Check sheet for the drawn part. Datum: minimum x, y, z corner. Units: mm. Give positions to 0.01 mm unless a question says otherwise; leave off trailing zeros. Loops run counter-clockwise (first coordinate to the right, second up) from the corner with the lowest first, then second, coordinate; pieces in that order, holes last.
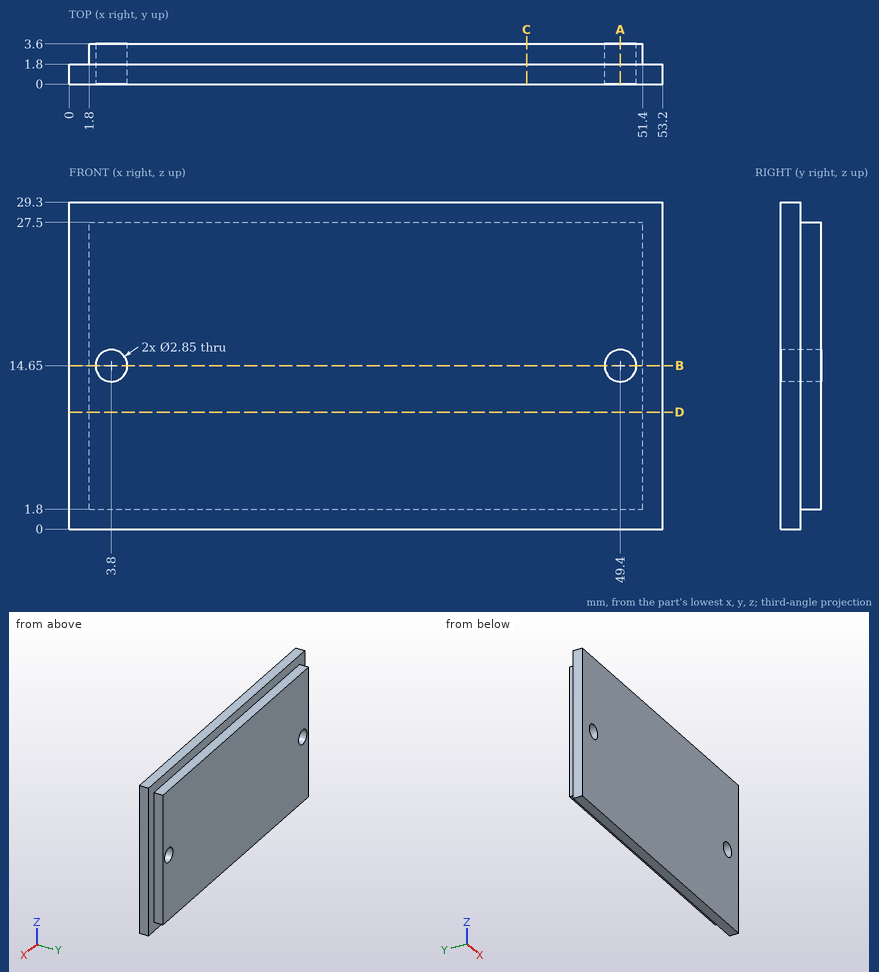
1) Sectioned sample at D-D on z = 10.5. Enter the section's corners in (x, y).
2) Sectioned sample at C-C on x = 41. Enter the section's corners in (y, z), plus the area to 3 significant figures.
3) Depth check by flat-ended pin: P1, Ø2.5, axis at x = 3.8, z = 14.65, coming from the -Y side (3 decimals); P2, Ø0.5, axis at y = 2.5, z = 14.5, coming from the -X side; P3, Ø2, axis at x = 37, y = 3, coming from the +Z side; P4, Ø1.4, axis at x = 38.5, y = 3, coming from the -Z side. Enter the tip coordinate at first touch or a pass-through.
4) Sectioned sample at A-A on x = 49.4. Enter the section's corners in (y, z) (3 decimals).
5) Sectioned sample at B-B on z = 14.65. Enter the section's corners in (x, y) (3 decimals).
6) Scan lines: line 1 along Z through (x, y) = (49.4, 1.7) (3 decimals); line 2 along X through (y, z) = (2.3, 10); line 3 along Z through (x, y) = (32.5, 2). Record each from-to range of solid material in increasing order.
Determined:
1. outline: (0, 0) - (53.2, 0) - (53.2, 1.8) - (51.4, 1.8) - (51.4, 3.6) - (1.8, 3.6) - (1.8, 1.8) - (0, 1.8) - close
2. outline: (0, 0) - (1.8, 0) - (1.8, 1.8) - (3.6, 1.8) - (3.6, 27.5) - (1.8, 27.5) - (1.8, 29.3) - (0, 29.3) - close
2. area: 99.0 mm2
3. P1: passes through
3. P2: stops at x = 1.8
3. P3: stops at z = 27.5
3. P4: stops at z = 1.8
4. outline: (0, 0) - (1.8, 0) - (1.8, 1.8) - (3.6, 1.8) - (3.6, 13.225) - (0, 13.225) - close; (0, 16.075) - (3.6, 16.075) - (3.6, 27.5) - (1.8, 27.5) - (1.8, 29.3) - (0, 29.3) - close
5. outline: (0, 0) - (2.375, 0) - (2.375, 3.6) - (1.8, 3.6) - (1.8, 1.8) - (0, 1.8) - close; (5.225, 0) - (47.975, 0) - (47.975, 3.6) - (5.225, 3.6) - close; (50.825, 0) - (53.2, 0) - (53.2, 1.8) - (51.4, 1.8) - (51.4, 3.6) - (50.825, 3.6) - close
6. line 1: z = 0 to 13.225, 16.075 to 29.3
6. line 2: x = 1.8 to 51.4
6. line 3: z = 1.8 to 27.5
